Build history of the part. All positions in model axes, mm. Face numbers are marked on the shaded views. A direction names the side the tool comes from. Coordinates: 2 decimals unless noted, no trailing zeros. Loops run counter-clockwise (first coordinate to the right, second up) from the corner with the lowest first, then second, coordinate; pieces in that order, holes last.
(1) Tool access for the marked faces 5, 6 and 7: list every direction of +Z, -Z, +X, -X, +Y, -Y with a clear straight run to the whole face (end or side of a thin tool).
(2) Flat gauge pins, fed straight in: P1, Ø2, axis at y = -4.5, z = 3, coming from the +X side; P2, Ø8.5, axis at x = 0, y = 0, coming from the -Z side; P3, Ø1.2, axis at x = -8, z = 3.5, coming from the +Y side; P4, Ø2.5, axis at x = 12.5, y = 0, coming from the +Z side. Where does each tip first touch, or does it go through?
(3) Wall check: L1, parallel to Y at x = 0, z = 1.55; L2, parallel to X at y = -2, z = 3.5; L3, parallel to X at y = -1.25, z = 2.4. Give the ranges that are in metal, low to high.
(4) Slice it at A-A (z = 0.45). Give the cut face in (x, y), and give its area (3 significant figures).
(5) Slice it at C-C (y = 0). Give the number of separate pieces and of enclosed holes in the cut face, and give its area (3 significant figures).
(6) Two-plate mould, pull along Y, no slides. Class the marked faces 1, 2, 3 and 4: pulls with the +Y half, pulls with the -Y half, needs draft (parallel to the pull), parting line crosses it, or undercut.
(7) Slice it at B-B (x = 0). Give the cut face in (y, z).
(8) Slice it at D-D (z = 4.6). Give the cut face in (x, y), and give its area (3 significant figures).
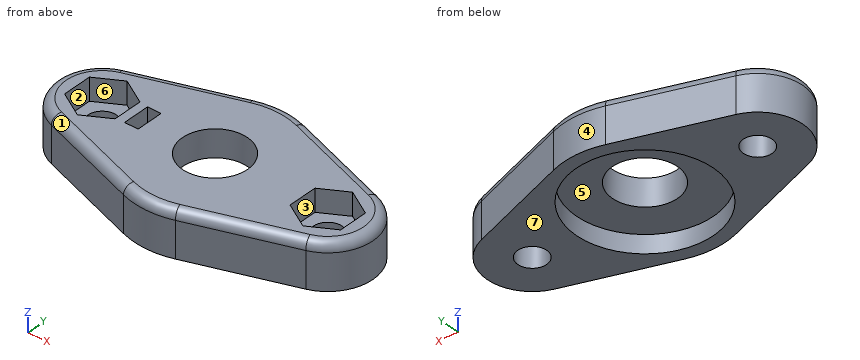
from build123d import *

# Parameters (mm, degrees)
EXTRUDE_1_DEPTH     = 5
SKETCH_1_3_R        = 7.6
CUT_EXTRUDE_1_DEPTH = 2
SKETCH_1_4_R        = 3.6
SKETCH_1_4_R_2      = 1.6
CUT_EXTRUDE_2_DEPTH = 5
CUT_EXTRUDE_START   = 5
SKETCH_1_5_W        = 1.5
SKETCH_1_5_H        = 3
CUT_EXTRUDE_3_DEPTH = 2.5
CUT_EXTRUDE_4_DEPTH = 2.5
FILLET_1_R          = 1


with BuildPart() as part:
    # Эскиз1 → Бобышка-Вытянуть1 (new body)
    with BuildSketch(Plane.XY):
        with BuildLine():
            Line((-14.1, 4.737087713), (-2.88, 8.526757883))
            ThreePointArc((-2.88, 8.526757883), (0, 9), (2.88, 8.526757883))
            Line((2.88, 8.526757883), (14.1, 4.737087713))
            ThreePointArc((14.1, 4.737087713), (17.5, 0), (14.1, -4.737087713))
            Line((14.1, -4.737087713), (2.88, -8.526757883))
            ThreePointArc((2.88, -8.526757883), (0, -9), (-2.88, -8.526757883))
            Line((-2.88, -8.526757883), (-14.1, -4.737087713))
            ThreePointArc((-14.1, -4.737087713), (-17.5, 0), (-14.1, 4.737087713))
        make_face()
    extrude(amount=EXTRUDE_1_DEPTH)

    # Эскиз1<3> → Вырез-Вытянуть1 (cut)
    with BuildSketch(Plane.XY):
        Circle(SKETCH_1_3_R)
    extrude(amount=CUT_EXTRUDE_1_DEPTH, mode=Mode.SUBTRACT)

    # Эскиз1<4> → Вырез-Вытянуть2 (cut)
    with BuildSketch(Plane.XY):
        Circle(SKETCH_1_4_R)
        with Locations((-12.5, 0)):
            Circle(SKETCH_1_4_R_2)
        with Locations((12.5, 0)):
            Circle(SKETCH_1_4_R_2)
    extrude(amount=CUT_EXTRUDE_2_DEPTH, mode=Mode.SUBTRACT)

    # Эскиз1<5> → Вырез-Вытянуть3 (cut)
    with BuildSketch(Plane.XY.offset(CUT_EXTRUDE_START)):
        with Locations((-8, 0)):
            Rectangle(SKETCH_1_5_W, SKETCH_1_5_H)
    extrude(amount=-CUT_EXTRUDE_3_DEPTH, mode=Mode.SUBTRACT)

    # Эскиз2 → Вырез-Вытянуть4 (cut)
    with BuildSketch(Plane.XY.offset(5)):
        Polygon((-12.5, 3.233161507), (-15.3, 1.616580754), (-15.3, -1.616580754), (-12.5, -3.233161507), (-9.7, -1.616580754), (-9.7, 1.616580754), align=None)
        Polygon((12.5, 3.233161507), (9.7, 1.616580754), (9.7, -1.616580754), (12.5, -3.233161507), (15.3, -1.616580754), (15.3, 1.616580754), align=None)
    extrude(amount=-CUT_EXTRUDE_4_DEPTH, mode=Mode.SUBTRACT)

    # Скругление1
    fillet_1_edges = [part.edges().sort_by_distance(p)[0] for p in [
        (0, -9, 5),
        (-8.49, -6.631922798, 5),
        (-17.5, 0, 5),
        (-8.49, 6.631922798, 5),
        (0, 9, 5),
        (8.49, 6.631922798, 5),
        (17.5, 0, 5),
        (8.49, -6.631922798, 5),
    ]]
    fillet(fillet_1_edges, radius=FILLET_1_R)


solid = part.part
Response values:
1. face 5: -Z
1. face 6: +Z
1. face 7: -Z, +X, -X, +Y, -Y
2. P1: stops at x = 16.07
2. P2: stops at z = 2
2. P3: stops at y = 7
2. P4: passes through
3. L1: y = -9 to -7.6, 7.6 to 9
3. L2: x = -17.08 to -14.64, -10.36 to -2.99, 2.99 to 10.36, 14.64 to 17.08
3. L3: x = -17.34 to -13.5, -11.5 to -3.38, 3.38 to 11.5, 13.5 to 17.34
4. outline: (-14.1, -4.74) - (-2.88, -8.53) arc R9 ccw to (2.88, -8.53) - (14.1, -4.74) arc R5 ccw to (14.1, 4.74) - (2.88, 8.53) arc R9 ccw to (-2.88, 8.53) - (-14.1, 4.74) arc R5 ccw to start; hole circle Ø3.2 at (-12.5, 0); hole circle Ø15.2 at (0, 0); hole circle Ø3.2 at (12.5, 0)
4. area: 249 mm2
5. separate pieces: 4
5. enclosed holes: 0
5. area: 74.8 mm2
6. face 1: pulls with the -Y half
6. face 2: undercut
6. face 3: undercut
6. face 4: pulls with the +Y half
7. outline: (-9, 0) - (-7.6, 0) - (-7.6, 2) - (-3.6, 2) - (-3.6, 5) - (-8, 5) arc R1 ccw to (-9, 4) - close; (3.6, 2) - (7.6, 2) - (7.6, 0) - (9, 0) - (9, 4) arc R1 ccw to (8, 5) - (3.6, 5) - close
8. outline: (-14.04, -4.55) - (-2.82, -8.34) arc R8.8 ccw to (2.82, -8.34) - (14.04, -4.55) arc R4.8 ccw to (14.04, 4.55) - (2.82, 8.34) arc R8.8 ccw to (-2.82, 8.34) - (-14.04, 4.55) arc R4.8 ccw to start; hole (-15.3, -1.62) - (-12.5, -3.23) - (-9.7, -1.62) - (-9.7, 1.62) - (-12.5, 3.23) - (-15.3, 1.62) - close; hole (-8.75, -1.5) - (-7.25, -1.5) - (-7.25, 1.5) - (-8.75, 1.5) - close; hole circle Ø7.2 at (0, 0); hole (9.7, -1.62) - (12.5, -3.23) - (15.3, -1.62) - (15.3, 1.62) - (12.5, 3.23) - (9.7, 1.62) - close
8. area: 330 mm2
